Here's how the part is built. I have some questions about the finished solid (model axes, mm). A direction names the side the tool comes from. Coordinates: 2 decimals unless noted, no trailing zeros. Order: outer loops, then holes, each group sorted by start corner. A loop starts at its lowest first (then second) coordinate and runs counter-clockwise, first axis right, second up. Notation, with made-up numbers: (-31.75, -32.5) - (20.25, -32.5) arc R13 cw to (20.25, -27.5) - close; hole circle Ø1 at (21.25, 12.5). An arc over 180 degrees is marked (long way). Answer as CSV lines item,"result". Start each with the question number.
Item 1: Imagine slicing it at C-C on x = -4. List the corners of the cut face in (y, z) for me, and give its area (3 significant figures).
Item 2: Imagine slicing it at B-B on y = 4. List the corners of the cut face in (x, z) for me, and give its area (3 significant figures).
Item 3: We'd pull the mould along Y, two halves only. Please class faces 1 (the face through (17, 0, -1)), 2 (the face through (25.43, 6.32, -0.99)), 3 (the face through (-1.19, -1.37, 1.04)), 4 (the face through (10, 4, -2)): pulls with the +Y half, pulls with the -Y half, needs draft (parallel to the pull), parting line crosses it, or undercut.
Item 4: Imagine slicing it at D-D on z = 2.5. List the corners of the cut face in (x, y) for me, and give its area (3 significant figures).
Item 5: I'm going to push flat-ended pins straight in: pin 1 (2 mm diameter, centred on x = 3, z = 0.5, fed in from +Y); pin 2 (3 mm diameter, centred on y = 6.5, z = 0.5, fed in from -X); pin 3 (9 mm diameter, centred on x = 20, y = 3.5, fed in from +Z); pin 4 (2.5 mm diameter, centred on x = 24.43, y = 2, fed in from -Z). Where does each tip first touch, or does it pass through?
Item 6: Imagine slicing it at A-A on x = 0. List the corners of the cut face in (y, z) for me.
Item 7: I need wall thicknesses on line 1 (Z direction, x = 22, y = 5.5); line 2 (Y direction, x = 14, z = -0.5); line 3 (Z direction, x = 0, y = 10.55). Which ranges of each line are inside material? Lowest first, please.
Item 8: On a 3-axis mill with a long thin cutter (end or side, diameter ignored), from which of +Z, -Z, +X, -X, +Y, -Y can I reach the whole of each face in a straight line? I mean faces 5 (the face through (4, 8, 4)), 6 (the face through (17, 8, -1)). Say none if no direction works.
from build123d import *

# Parameters (mm, degrees)
BOSS_EXTRUDE1_DEPTH     = 8
SKETCH6_R               = 7.5
BOSS_EXTRUDE3_DEPTH     = 6
SKETCH2_R               = 5.5
CUT_EXTRUDE4_DEPTH      = 5
CUT_EXTRUDE4_DEPTH_BACK = 3
SKETCH8_R               = 0.8
CUT_EXTRUDE5_DEPTH      = 16
FILLET3_R               = 3
SKETCH9_R               = 1.05
CUT_EXTRUDE6_DEPTH      = 3.0000001


with BuildPart() as part:
    # Sketch1 → Boss-Extrude1 (new body)
    with BuildSketch(Plane(origin=(0, 0, 0), x_dir=(1, 0, 0), z_dir=(0, 1, 0))):
        Polygon((0, 0), (0, 2), (26.334414729, 2), (27.267030045, 0), (21.996962058, 0), align=None)
    extrude(amount=BOSS_EXTRUDE1_DEPTH)

    # Sketch6 → Boss-Extrude3 (add)
    with BuildSketch(Plane(origin=(0, 0, -2), x_dir=(-1, 0, 0), z_dir=(0, 0, -1))):
        with Locations((0, 4)):
            Circle(SKETCH6_R)
    extrude(amount=-BOSS_EXTRUDE3_DEPTH)

    # Sketch2 → Cut-Extrude4 (cut, two sides)
    with BuildSketch(Plane.XY) as cut_extrude4_sk:
        with Locations((0, 4)):
            Circle(SKETCH2_R)
    extrude(amount=CUT_EXTRUDE4_DEPTH, mode=Mode.SUBTRACT)
    extrude(cut_extrude4_sk.sketch, amount=-CUT_EXTRUDE4_DEPTH_BACK, mode=Mode.SUBTRACT)

    # Sketch8 → Cut-Extrude5 (cut, through all)
    with BuildSketch(Plane(origin=(0, -3.5, 0), x_dir=(-1, 0, 0), z_dir=(0, -1, 0))):
        with Locations((0, -1.034043254)):
            Circle(SKETCH8_R)
    extrude(amount=-CUT_EXTRUDE5_DEPTH, mode=Mode.SUBTRACT)

    # Fillet3
    fillet3_edges = [part.edges().sort_by_distance(p)[0] for p in [
        (7.5, 4, 0),
    ]]
    fillet(fillet3_edges, radius=FILLET3_R)

    # Sketch9 → Cut-Extrude6 (cut, through all)
    with BuildSketch(Plane.XY):
        with Locations((24.429577374, 2)):
            Circle(SKETCH9_R)
        with Locations((24.429577374, 6)):
            Circle(SKETCH9_R)
    extrude(amount=-CUT_EXTRUDE6_DEPTH, mode=Mode.SUBTRACT)


solid = part.part
Responses:
1,outline,"(-2.34, -2) - (0.23, -2) - (0.23, 4) - (-2.34, 4) - close; (7.77, -2) - (10.34, -2) - (10.34, 4) - (7.77, 4) - close"
1,area,"30.8 mm^2"
2,outline,"(-7.5, -2) - (-5.5, -2) - (-5.5, 4) - (-7.5, 4) - close; (5.5, -2) - (26.33, -2) - (27.27, 0) - (10.5, 0) arc R3 cw to (7.5, 3) - (7.5, 4) - (5.5, 4) - close"
2,area,"64.5 mm^2"
3,face 1,"pulls with the -Y half"
3,face 2,"undercut"
3,face 3,"undercut"
3,face 4,"needs draft"
4,outline,"(6.34, 0) - (6.39, 0) arc R7.54 ccw to (6.39, 8) - (6.34, 8) arc R7.5 ccw (long way) to start; hole circle Ø11 at (0, 4)"
4,area,"82.0 mm^2"
5,pin 1,"stops at y = 11.23"
5,pin 2,"stops at x = -7.43"
5,pin 3,"stops at z = 0"
5,pin 4,"stops at z = -2"
6,outline,"(-3.5, -2) - (-1.5, -2) - (-1.5, 0.23) - (-3.5, 0.23) - close; (-3.5, 1.83) - (-1.5, 1.83) - (-1.5, 4) - (-3.5, 4) - close; (9.5, -2) - (11.5, -2) - (11.5, 0.23) - (9.5, 0.23) - close; (9.5, 1.83) - (11.5, 1.83) - (11.5, 4) - (9.5, 4) - close"
7,line 1,"z = -2 to 0"
7,line 2,"y = 0 to 8"
7,line 3,"z = -2 to 0.23, 1.83 to 4"
8,face 5,"+Z, +X, -X, +Y, -Y"
8,face 6,"+Z, -Z, +X, +Y"
